from build123d import *

# Parameters (mm, degrees)
CROQUIS1_W              = 180
CROQUIS1_H              = 180
SALIENTE_EXTRUIR1_DEPTH = 30.7
CROQUIS2_W              = 162.99
CROQUIS2_H              = 162.21
CORTAR_EXTRUIR1_DEPTH   = 20.7
CROQUIS4_W              = 175
CROQUIS4_H              = 10.7
CORTAR_EXTRUIR2_DEPTH   = 175
CROQUIS5_W              = 40
CROQUIS5_H              = 38
CORTAR_EXTRUIR3_DEPTH   = 10
CROQUIS6_W              = 82.99
CROQUIS6_H              = 38
CORTAR_EXTRUIR4_DEPTH   = 5
CROQUIS7_W              = 10
CROQUIS7_H              = 97.21
CORTAR_EXTRUIR5_DEPTH   = 5
CROQUIS8_W              = 10
CROQUIS8_H              = 30
CORTAR_EXTRUIR6_DEPTH   = 20
CROQUIS9_R              = 1.4
CORTAR_EXTRUIR7_DEPTH   = 20
CHAFL_N1_SIZE           = 15
CHAFL_N1_SIZE2          = 8.660254038


with BuildPart() as part:
    # Croquis1 → Saliente-Extruir1 (new body)
    with BuildSketch(Plane.XY):
        with Locations((90, 90)):
            Rectangle(CROQUIS1_W, CROQUIS1_H)
    extrude(amount=SALIENTE_EXTRUIR1_DEPTH)

    # Croquis2 → Cortar-Extruir1 (cut)
    with BuildSketch(Plane(origin=(0, 0, 0), x_dir=(-1, 0, 0), z_dir=(0, 0, -1))):
        with Locations((-98.505, 98.895)):
            Rectangle(CROQUIS2_W, CROQUIS2_H)
    extrude(amount=-CORTAR_EXTRUIR1_DEPTH, mode=Mode.SUBTRACT)

    # Croquis4 → Cortar-Extruir2 (cut)
    with BuildSketch(Plane(origin=(0, 180, 0), x_dir=(1, 0, 0), z_dir=(0, 1, 0))):
        with Locations((92.5, -15.35)):
            Rectangle(CROQUIS4_W, CROQUIS4_H)
    extrude(amount=-CORTAR_EXTRUIR2_DEPTH, mode=Mode.SUBTRACT)

    # Croquis5 → Cortar-Extruir3 (cut)
    with BuildSketch(Plane(origin=(0, 0, 20.7), x_dir=(-1, 0, 0), z_dir=(0, 0, -1))):
        with Locations((-160, 161)):
            Rectangle(CROQUIS5_W, CROQUIS5_H)
        with Locations((-37.01, 161)):
            Rectangle(CROQUIS5_W, CROQUIS5_H)
    extrude(amount=-CORTAR_EXTRUIR3_DEPTH, mode=Mode.SUBTRACT)

    # Croquis6 → Cortar-Extruir4 (cut)
    with BuildSketch(Plane.XY.offset(30.7)):
        with Locations((98.505, 161)):
            Rectangle(CROQUIS6_W, CROQUIS6_H)
    extrude(amount=-CORTAR_EXTRUIR4_DEPTH, mode=Mode.SUBTRACT)

    # Croquis7 → Cortar-Extruir5 (cut)
    with BuildSketch(Plane(origin=(0, 0, 20.7), x_dir=(-1, 0, 0), z_dir=(0, 0, -1))):
        with Locations((-175, 66.395)):
            Rectangle(CROQUIS7_W, CROQUIS7_H)
    extrude(amount=-CORTAR_EXTRUIR5_DEPTH, mode=Mode.SUBTRACT)

    # Croquis8 → Cortar-Extruir6 (cut)
    with BuildSketch(Plane(origin=(0, 0, 20.7), x_dir=(-1, 0, 0), z_dir=(0, 0, -1))):
        with Locations((-10, 20)):
            Rectangle(CROQUIS8_W, CROQUIS8_H)
    extrude(amount=-CORTAR_EXTRUIR6_DEPTH, mode=Mode.SUBTRACT)

    # Croquis9 → Cortar-Extruir7 (cut)
    with BuildSketch(Plane(origin=(0, 0, 20.7), x_dir=(-1, 0, 0), z_dir=(0, 0, -1))):
        with Locations((-120, 161)):
            Circle(CROQUIS9_R)
        with Locations((-77.01, 161)):
            Circle(CROQUIS9_R)
        with Locations((-175, 95)):
            Circle(CROQUIS9_R)
        with Locations((-175, 37.79)):
            Circle(CROQUIS9_R)
    extrude(amount=-CORTAR_EXTRUIR7_DEPTH, mode=Mode.SUBTRACT)

    # Chaflán1
    chafl_n1_edges = [part.edges().sort_by_distance(p)[0] for p in [
        (98.505, 17.79, 0),
        (17.01, 98.895, 0),
    ]]
    chafl_n1_side = [part.faces().sort_by_distance(p)[0] for p in [
        (2.545584412, 90, 0),
    ]]
    chamfer(chafl_n1_edges, length=CHAFL_N1_SIZE, length2=CHAFL_N1_SIZE2, reference=chafl_n1_side[0])


solid = part.part
Model file for the job. Use its own axes, mm. A direction names the side the tool comes from. Coordinates: 2 decimals unless noted, no trailing zeros. Order: outer loops, then holes, each group sorted by start corner. A loop starts at its lowest first (then second) coordinate and runs counter-clockwise, first axis right, second up. Notation, with made-up numbers: (-2.75, 61.25) -> (5.25, 61.25) arc R28 ccw to (5.25, 88.25) -> close; hole circle Ø8 at (33.25, -39). An arc over 180 degrees is marked (long way). Return JSON: item names as keys, results as strings. Group by question number.
Item 1: Saw through at D-D on z = 5. Write the cut outline in (x, y), then the cut area to 3 significant figures.
Item 2: Wall check: line 1 along Y through (x, z) = (175, 29.15); line 2 along X through (y, z) = (161, 24); line 3 along X through (y, z) = (95, 28.75). Give the ranges that are in metal, low to high. Write a range as [from, to].
Item 3: Pull direction Y, two halves, no side cores. Call faces 5 (the flat face through (98, 180, 23)), 6 (the flat face through (9.61, 90.15, 4.39)), 7 (the flat face through (175, 17.79, 23)): pulls with the +Y half, pulls with the -Y half, needs draft (parallel to the pull), parting line crosses it, or undercut.
Item 4: Saw through at A-A on x = 113. Write the cut outline in (y, z).
Item 5: Saw through at C-C on y = 123. Write the cut outline in (x, z), then the cut area to 3 significant figures.
Item 6: Saw through at B-B on z = 23. Write the cut outline in (x, y).
Item 7: Tool access for faces 1 (the flat face through (15, 20, 26)), 2 (the flat face through (140, 161, 23)), 3 (the flat face through (98, 161, 25.7)), 4 (the flat face through (91, 94, 20.7)): list every direction of +Z, -Z, +X, -X, +Y, -Y with a clear straight run to the whole face (end or side of a thin tool).
Item 8: Flat gauge pins, fed straight in: P1, Ø11, axis at x = 176, y = 50, coming from the -Z side; P2, Ø1.5, axis at x = 90.5, z = 20.5, coming from the -Y side; P3, Ø2.5, axis at x = 77.01, y = 161, coming from the +Z side; P4, Ø1.5, axis at x = 172.5, z = 24, coming from the +Y side. Where does each tip first touch, or does it go through?
Values found:
{
 "1": {"outline": "(0, 0) -> (180, 0) -> (180, 11.45) -> (10.67, 11.45) -> (10.67, 180) -> (0, 180) -> close", "area": "3,860 mm2"},
 "2": {"line 1": "y = [0, 36.39], [39.19, 93.6], [96.4, 142]", "line 2": "x = [0, 17.01], [57.01, 75.61], [78.41, 118.6], [121.4, 140]", "line 3": "x = [0, 173.6], [176.4, 180]"},
 "3": {"face 5": "pulls with the +Y half", "face 6": "needs draft", "face 7": "undercut"},
 "4": {"outline": "(0, 0) -> (2.79, 0) -> (17.79, 8.66) -> (17.79, 10) -> (5, 10) -> (5, 20.7) -> (180, 20.7) -> (180, 25.7) -> (142, 25.7) -> (142, 30.7) -> (0, 30.7) -> close"},
 "5": {"outline": "(0, 0) -> (2.01, 0) -> (17.01, 8.66) -> (17.01, 10) -> (5, 10) -> (5, 20.7) -> (180, 20.7) -> (180, 30.7) -> (0, 30.7) -> close", "area": "1,960 mm2"},
 "6": {"outline": "(0, 0) -> (180, 0) -> (180, 17.79) -> (170, 17.79) -> (170, 115) -> (180, 115) -> (180, 142) -> (140, 142) -> (140, 180) -> (57.01, 180) -> (57.01, 142) -> (17.01, 142) -> (17.01, 180) -> (0, 180) -> close; hole (5, 5) -> (15, 5) -> (15, 35) -> (5, 35) -> close; hole circle Ø2.8 at (77.01, 161); hole circle Ø2.8 at (120, 161)"},
 "7": {"face 1": "+Z", "face 2": "+Z, -Z, +X, +Y", "face 3": "+Z, +X, +Y", "face 4": "+X, +Y"},
 "8": {"P1": "stops at z = 25.7", "P2": "stops at y = 0", "P3": "passes through", "P4": "stops at y = 142"}
}
